from build123d import *

# Parameters (mm, degrees)
F0_R     = 0.968937
F0_R_2   = 0.293951
F0_R_3   = 4.095338
F1_DEPTH = 0.2794


with BuildPart() as f1:
    # F0 (on Top) → F1 (new body)
    with BuildSketch(Plane.XY):
        with BuildLine():
            ThreePointArc((4.330335, -5.676164), (6.006943, -6.368025), (7.110444, -4.928592))
            ThreePointArc((7.110444, -4.928592), (6.899941, -4.164898), (6.327886, -3.616909))
            ThreePointArc((6.327886, -3.616909), (4.549982, -3.890753), (4.330335, -5.676164))
        make_face()
        with Locations((5.619878, -4.928592)):
            Circle(F0_R, mode=Mode.SUBTRACT)
        with BuildLine():
            ThreePointArc((4.330335, -5.676164), (4.549982, -3.890753), (6.327886, -3.616909))
            ThreePointArc((6.327886, -3.616909), (5.018305, -0.522851), (6.7365, 2.364362))
            ThreePointArc((6.7365, 2.364362), (5.106348, 3.124981), (5.395309, 4.900491))
            ThreePointArc((5.395309, 4.900491), (2.048002, 4.611122), (-0.166949, 7.13742))
            ThreePointArc((-0.166949, 7.13742), (-1.394085, 5.822098), (-2.993402, 6.645579))
            ThreePointArc((-2.993402, 6.645579), (-3.75257, 3.372681), (-6.83968, 2.046806))
            ThreePointArc((-6.83968, 2.046806), (-6.194158, 1.496962), (-5.952965, 0.684033))
            ThreePointArc((-5.952965, 0.684033), (-6.321654, -0.297385), (-7.245333, -0.793298))
            ThreePointArc((-7.245333, -0.793298), (-4.367218, -2.52669), (-4.060206, -5.872425))
            ThreePointArc((-4.060206, -5.872425), (-2.417795, -5.475804), (-1.460165, -6.867841))
            ThreePointArc((-1.460165, -6.867841), (-1.466251, -7.002402), (-1.48446, -7.135864))
            ThreePointArc((-1.48446, -7.135864), (1.05348, -4.934261), (4.330335, -5.676164))
        make_face()
        with Locations((-3.970255, -2.362004)):
            Circle(F0_R_2, mode=Mode.SUBTRACT)
        with Locations((1.019524, -4.505836)):
            Circle(F0_R_2, mode=Mode.SUBTRACT)
        Circle(F0_R_3, mode=Mode.SUBTRACT)
        with Locations((4.600355, -0.422755)):
            Circle(F0_R_2, mode=Mode.SUBTRACT)
        with Locations((-3.473276, 3.046037)):
            Circle(F0_R_2, mode=Mode.SUBTRACT)
        with Locations((1.823652, 4.244559)):
            Circle(F0_R_2, mode=Mode.SUBTRACT)
        with BuildLine():
            ThreePointArc((5.395309, 4.900491), (5.106348, 3.124981), (6.7365, 2.364362))
            ThreePointArc((6.7365, 2.364362), (7.583226, 2.884788), (7.914573, 3.821803))
            ThreePointArc((7.914573, 3.821803), (7.010712, 5.192046), (5.395309, 4.900491))
        make_face()
        with Locations((6.424007, 3.821803)):
            Circle(F0_R, mode=Mode.SUBTRACT)
        with BuildLine():
            ThreePointArc((-4.060206, -5.872425), (-3.607157, -8.206082), (-1.48446, -7.135864))
            ThreePointArc((-1.48446, -7.135864), (-1.466251, -7.002402), (-1.460165, -6.867841))
            ThreePointArc((-1.460165, -6.867841), (-2.417795, -5.475804), (-4.060206, -5.872425))
        make_face()
        with Locations((-2.950731, -6.867841)):
            Circle(F0_R, mode=Mode.SUBTRACT)
        with BuildLine():
            ThreePointArc((-2.993402, 6.645579), (-1.394085, 5.822098), (-0.166949, 7.13742))
            ThreePointArc((-0.166949, 7.13742), (-0.161032, 7.213907), (-0.159058, 7.290596))
            ThreePointArc((-0.159058, 7.290596), (-1.980378, 8.744002), (-2.993402, 6.645579))
        make_face()
        with Locations((-1.649624, 7.290596)):
            Circle(F0_R, mode=Mode.SUBTRACT)
        with BuildLine():
            ThreePointArc((-6.83968, 2.046806), (-8.919121, 0.894792), (-7.245333, -0.793298))
            ThreePointArc((-7.245333, -0.793298), (-6.321654, -0.297385), (-5.952965, 0.684033))
            ThreePointArc((-5.952965, 0.684033), (-6.194158, 1.496962), (-6.83968, 2.046806))
        make_face()
        with Locations((-7.443531, 0.684033)):
            Circle(F0_R, mode=Mode.SUBTRACT)
    extrude(amount=F1_DEPTH)


solid = f1.part
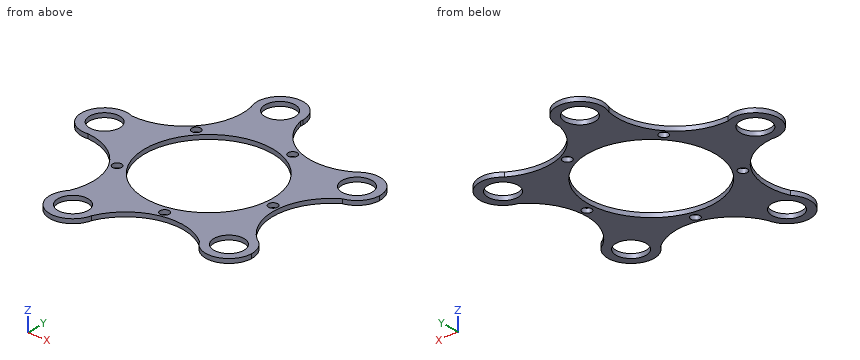
Model file for the job. Use its own axes, mm. Round coordinates to 2 decimals unless told otherwise and drop trailing zeros. Order: outer loops, then holes, each group sorted by start corner. A loop starts at its lowest first (then second) coordinate and runs counter-clockwise, first axis right, second up. Notation, with made-up numbers: M -4.5,61 L -0.5,61 A36 ccw -0.5,97 Z; hole C 59,-40 d7. An arc over 180 degrees is marked long. Write each question's results on one line, items separated by ' | '. Start each with the question number.
(1) Saw through at B-B, the plane z = 0.2. State how many separate pieces and enclosed holes the cut face has, then the cut area to 3 significant figures.
(2) Probe probe 1 along Y at (x, z) = (-1, 0.15); probe 2 along X at (y, z) = (-4.5, 0.1); probe 3 along Y at (x, z) = (5.75, 0.2). List the from-to ranges inside material, lowest first. Write a range as from..to.
(3) Drop a flat-ended pin along its axis: pin 1 (1.6 mm diameter, centred on x = 5.62, y = -4.93, fed in from -Z). Give the stop position or say it passes through.
(4) Saw through at A-A, the plane x = 2.75. Give the cut face in (y, z), then the cut area to 3 significant figures.
Established:
1) separate pieces: 1 | enclosed holes: 11 | area: 71.7 mm^2
2) probe 1: y = -6.29..-3.97, 3.97..6.57, 8.01..8.63 | probe 2: x = -3.8..0.73, 1.31..4.75, 6.49..7.05 | probe 3: y = -6.41..-5.89, -3.97..-3, 1.45..3.13, 4.52..5.15
3) pin 1: passes through
4) outline: M -4.91,0 L -3.03,0 L -3.03,0.28 L -4.91,0.28 Z; M 3.03,0 L 4.41,0 L 4.41,0.28 L 3.03,0.28 Z | area: 0.906 mm^2
